```python
from build123d import *

# Parameters (mm, degrees)
F1_DEPTH = 914.4


with BuildPart() as f1:
    # F0 (on Top) → F1 (new body)
    with BuildSketch(Plane.XY):
        with BuildLine():
            Line((442.876746, -496.589411), (0, 0))
            Line((0, 0), (-442.876746, -496.589411))
            ThreePointArc((-442.876746, -496.589411), (-493.663388, -583.230539), (-507.080321, -682.759199))
            ThreePointArc((-507.080321, -682.759199), (-504.622043, -684.893954), (-502.518043, -682.409302))
            ThreePointArc((-502.518043, -682.409302), (-490.069762, -584.357788), (-437.834835, -500.449675))
            Line((-437.834835, -500.449675), (0, -50.8))
            Line((0, -50.8), (437.834835, -500.449675))
            ThreePointArc((437.834835, -500.449675), (490.069762, -584.357788), (502.518043, -682.409302))
            ThreePointArc((502.518043, -682.409302), (504.622043, -684.893954), (507.080321, -682.759199))
            ThreePointArc((507.080321, -682.759199), (493.663388, -583.230539), (442.876746, -496.589411))
        make_face()
    extrude(amount=F1_DEPTH)


solid = f1.part
```
CAD build for the part. Positions are in the model's coordinates, mm. A direction names the side the tool comes from. Coordinates: 2 decimals unless noted, no trailing zeros. Loops run counter-clockwise (first coordinate to the right, second up) from the corner with the lowest first, then second, coordinate; pieces in that order, holes last. Notation, with made-up numbers: (6, 77) - (64, 77) arc R17 ccw to (64, 82) - close; hole circle Ø9 at (-21.75, 87). An arc over 180 degrees is marked (long way). Use CSV: the item, a comma, the result in double quotes. Start each with the question number.
Q1. Cut at B-B, the plane y = -191.5. List the corners of the cut face in (x, z).
Q2. Probe probe 1 along X at (y, z) = (-256.5, 224.5); probe 2 along X at (y, z) = (-117.5, 626); probe 3 along Y at (x, z) = (101.5, 107). List the from-to ranges inside material, lowest first. Write a range as from..to.
Q3. Cut at D-D, the plane x = 315. List the corners of the cut face in (y, z).
Q4. Two-plate mould, pull along X, no slides. Class faces 1 (the flat face through (224.54, -251.77, 450.8)), 2 (the cylindrical face through (-490.53, -585.67, 450.8)), 3 (the flat face through (-218.34, -244.82, 450.8)), 4 (the flat face through (-221.98, -278.77, 450.8)): +X half, -X half, draft (parallel to the pull), parting line (faces both ways), or undercut.
Q5. Cut at A-A, the plane y = -340. List the corners of the cut face in (x, z), then the cut area to 3 significant figures.
Q6. Drop flat-ended pins along their axis: P1, Ø5, axis at x = 92.5, z = 430.5, coming from the -Y side; P2, Ø2, axis at x = 19.5, z = 203.5, coming from the -Y side; P3, Ø5, axis at y = -74, z = 159, coming from the +X side. Give the stop position or say it passes through.
Q7. 3-axis set-ups, long thin cutter, end or side, ignore diameter. For faces 5 (the cylindrical face through (489.6, -583.05, 450.8)), 6 (the flat face through (110, -163, 914.4)), 7 (the flat face through (215.853, -272.477, 450.799)): which of +Z, -Z, +X, -X, +Y, -Y reach the whole face in a straight line?
Q8. Cut at C-C, the plane z = 106. List the corners of the cut face in (x, y), then the cut area to 3 significant figures.
Here are the results:
1,outline,"(-170.79, 0) - (-137, 0) - (-137, 914.4) - (-170.79, 914.4) - close; (137, 0) - (170.79, 0) - (170.79, 914.4) - (137, 914.4) - close"
2,probe 1,"-228.76..-200.3, 200.3..228.76"
2,probe 2,"-104.79..-64.95, 64.95..104.79"
2,probe 3,"-155.04..-113.81"
3,outline,"(-374.3, 0) - (-353.2, 0) - (-353.2, 914.4) - (-374.3, 914.4) - close"
4,face 1,"+X half"
4,face 2,"undercut"
4,face 3,"-X half"
4,face 4,"undercut"
5,outline,"(-303.22, 0) - (-281.6, 0) - (-281.6, 914.4) - (-303.22, 914.4) - close; (281.6, 0) - (303.22, 0) - (303.22, 914.4) - (281.6, 914.4) - close"
5,area,"39,500 mm2"
6,P1,"y = -148.36"
6,P2,"y = -71.85"
6,P3,"x = 68.23"
7,face 5,"+Z, -Z"
7,face 6,"+Z, +X, -X, +Y, -Y"
7,face 7,"+Z, -Z, -Y"
8,outline,"(-507.08, -682.76) arc R2.29 ccw (long way) to (-502.52, -682.41) arc R231.35 cw to (-437.83, -500.45) - (0, -50.8) - (437.83, -500.45) arc R231.35 cw to (502.52, -682.41) arc R2.29 ccw (long way) to (507.08, -682.76) arc R255.15 ccw to (442.88, -496.59) - (0, 0) - (-442.88, -496.59) arc R255.15 ccw to start"
8,area,"28,200 mm2"
